Here's how the part is built. I have some questions about the finished solid (model axes, mm). A direction names the side the tool comes from. Round coordinates to 2 decimals unless told otherwise and drop trailing zeros. Order: outer loops, then holes, each group sorted by start corner. A loop starts at its lowest first (then second) coordinate and runs counter-clockwise, first axis right, second up. Notation, with made-up numbers: (-12, -8) -> (19, -8) arc R28 ccw to (19, 14) -> close; hole circle Ø2 at (-3, -2.75). An arc over 180 degrees is marked (long way). Use a Markdown table: item, result. Add a question column.
(1) I'm going to push flat-ended pins straight in: P1, Ø12, axis at x = 16, y = -123, coming from the +Z side; P2, Ø4, axis at x = -74.5, z = 42.5, coming from the -Y side; P3, Ø9, axis at y = -137, z = 9.5, coming from the -X side. Where does each tip first touch, or does it pass through?
(2) I want a section at B-B, the plane x = 28. Please give me the cut outline in (y, z).
(3) I want a section at C-C, the plane z = 27. Please give me the cut outline in (x, y), then the cut area to 3 significant figures.
(4) Thinking about a two-plate mould opening in X: for faces 1 (the face through (1, -121, 4)), 2 (the face through (1, -139, 12.5)), 3 (the face through (-28.334, -121, 14)), 4 (the face through (-20.334, -139, 8)), which applies, pulls with the +X half, pulls with the -X half, needs draft (parallel to the pull), parting line crosses it, or undercut?
(5) On a 3-axis mill with a long thin cutter (end or side, diameter ignored), from which of +Z, -Z, +X, -X, +Y, -Y can I reach the whole of each face in a straight line? I mean faces 5 (the face through (1, 4, 0)), 6 (the face through (1, -111, 12.5)), 7 (the face through (3.75, -128.505, 4.15)). Say none if no direction works.
(6) I want a section at D-D, the plane y = -104. Please give me the cut outline in (x, z), then the cut area to 3 significant figures.
(7) I want a section at A-A, the plane x = 0. Please give me the cut outline in (y, z), then the cut area to 3 significant figures.
(8) If I drill on probe 1 along X at (y, z) = (-136.5, 11.5); probe 2 along Z at (x, y) = (-22.5, -99.5); probe 3 along Y at (x, z) = (22, 34), over which ranges is the centre line in solid material (lowest first)?
from build123d import *

# Parameters (mm, degrees)
SKETCH1_R           = 98.505410199
BOSS_EXTRUDE1_DEPTH = 50
BOSS_EXTRUDE2_START = -5.228497
SKETCH2_W           = 60
SKETCH2_H           = 17
BOSS_EXTRUDE2_DEPTH = 55.228497
SKETCH3_W           = 44
SKETCH3_H           = 8
CUT_EXTRUDE1_DEPTH  = 40
SKETCH4_W           = 9
SKETCH4_H           = 15
CUT_EXTRUDE2_DEPTH  = 127.839445164


with BuildPart() as part:
    # Sketch1 → Boss-Extrude1 (new body)
    with BuildSketch(Plane.XY):
        Circle(SKETCH1_R)
    extrude(amount=BOSS_EXTRUDE1_DEPTH)

    # Sketch2 → Boss-Extrude2 (add)
    with BuildSketch(Plane(origin=(0, -98.505410199, 0), x_dir=(-1, 0, 0), z_dir=(0, -1, 0)).offset(BOSS_EXTRUDE2_START)):
        with Locations((-1.665965035, -8.5)):
            Rectangle(SKETCH2_W, SKETCH2_H)
    extrude(amount=BOSS_EXTRUDE2_DEPTH)

    # Sketch3 → Cut-Extrude1 (cut)
    with BuildSketch(Plane.XZ.offset(148.505410199)):
        with Locations((1.665965035, 8.5)):
            Rectangle(SKETCH3_W, SKETCH3_H)
    extrude(amount=-CUT_EXTRUDE1_DEPTH, mode=Mode.SUBTRACT)

    # Sketch4 → Cut-Extrude2 (cut, through all)
    with BuildSketch(Plane.ZY.offset(28.334034965)):
        with Locations((8.5, -121.005410199)):
            Rectangle(SKETCH4_W, SKETCH4_H)
    extrude(amount=-CUT_EXTRUDE2_DEPTH, mode=Mode.SUBTRACT)


solid = part.part
Taken from the geometry:
| question | item | result |
|---|---|---|
| 1 | P1 | stops at z = 17 |
| 1 | P2 | stops at y = -66.69 |
| 1 | P3 | stops at x = -28.33 |
| 2 | outline | (-148.51, 0) -> (94.44, 0) -> (94.44, 50) -> (-94.44, 50) -> (-94.44, 17) -> (-148.51, 17) -> close; hole (-128.51, 4) -> (-113.51, 4) -> (-113.51, 13) -> (-128.51, 13) -> close |
| 3 | outline | circle Ø197.01 at (0, 0) |
| 3 | area | 30,500 mm2 |
| 4 | face 1 | needs draft |
| 4 | face 2 | undercut |
| 4 | face 3 | pulls with the -X half |
| 4 | face 4 | undercut |
| 5 | face 5 | -Z, +X, -X, +Y, -Y |
| 5 | face 6 | -Y |
| 5 | face 7 | +X, -X |
| 6 | outline | (-28.33, 0) -> (31.67, 0) -> (31.67, 17) -> (-28.33, 17) -> close |
| 6 | area | 1,020 mm2 |
| 7 | outline | (-148.51, 0) -> (98.51, 0) -> (98.51, 50) -> (-98.51, 50) -> (-98.51, 17) -> (-148.51, 17) -> (-148.51, 12.5) -> (-128.51, 12.5) -> (-128.51, 13) -> (-113.51, 13) -> (-113.51, 12.5) -> (-108.51, 12.5) -> (-108.51, 4.5) -> (-113.51, 4.5) -> (-113.51, 4) -> (-128.51, 4) -> (-128.51, 4.5) -> (-148.51, 4.5) -> close |
| 7 | area | 10,400 mm2 |
| 8 | probe 1 | x = -28.33 to -20.33, 23.67 to 31.67 |
| 8 | probe 2 | z = 0 to 17 |
| 8 | probe 3 | y = -96.02 to 96.02 |
